```python
from build123d import *

# Parameters (mm, degrees)
SKETCH1_R           = 3.175
BOSS_EXTRUDE1_DEPTH = 2.54


with BuildPart() as part:
    # Sketch1 → Boss-Extrude1 (new body)
    with BuildSketch(Plane.XY):
        with BuildLine():
            Line((-0.792713517, -6.209589215), (80.497230298, -16.587028851))
            Line((80.497230298, -16.587028851), (106.74595178, -3.93139528))
            Line((106.74595178, -3.93139528), (106.274352446, 204.184578368))
            ThreePointArc((106.274352446, 204.184578368), (100.014368984, 210.444561829), (93.754385523, 204.184578368))
            Line((93.754385523, 204.184578368), (94.208186896, 3.92281412))
            Line((94.208186896, 3.92281412), (78.402076612, -3.697989053))
            Line((78.402076612, -3.697989053), (0.792713517, 6.209589215))
            ThreePointArc((0.792713517, 6.209589215), (-6.209589215, 0.792713517), (-0.792713517, -6.209589215))
        make_face()
        Circle(SKETCH1_R, mode=Mode.SUBTRACT)
        with Locations((100.014368984, 204.184578368)):
            Circle(SKETCH1_R, mode=Mode.SUBTRACT)
    extrude(amount=BOSS_EXTRUDE1_DEPTH)


solid = part.part
```
Source: CAD feature listing. Evaluate the final solid. Frame: model axes, mm. Coordinates: 2 decimals unless noted, no trailing zeros. Order: outer loops, then holes, each group sorted by start corner. A loop starts at its lowest first (then second) coordinate and runs counter-clockwise, first axis right, second up. Notation, with made-up numbers: M 88,-23.75 L 137,-23.75 A11 ccw 137,-13.75 Z; hole C -17.75,51.5 d5. An arc over 180 degrees is marked long. Write each question's results on one line, items separated by ' | '. Start each with the question number.
1) Section query B-B (y = 0). Return the cut outline in (x, z) (1 decimal), plus the area to 3 significant figures.
2) Section query C-C (x = 85.5). Return the cut outline in (y, z), plus the area to 3 significant figures.
3) Contact query for a flat-ended pin moving along its axis: pin 1 Ø1.5 at (x, z) = (17.5, 1) entering from +Y. Output: stop coordinate, or through.
4) Line query: line 1 (Y direction, x = 0, z = 1.45) (3 decimals); line 2 (X direction, y = 199, z = 0.7); line 3 (X direction, y = 13.5, z = 0.7). Output: solid intervals per line, ascending. Write a range as from..to.
5) Section query A-A (z = 1.15). Return the cut outline in (x, y) (3 decimals).
6) Draft query along Y for faces 1 (the face through (39.283, -11.326, 1.252)), 2 (the face through (-0.69, -3.1, 1.25)), 3 (the face through (40.141, 1.186, 1.252)). Return one class per face: released by +Y, released by -Y, zero draft, split by the parting line, or undercut.
7) Section query D-D (y = 172). Return the cut outline in (x, z).
Answers:
1) outline: M -6.3,0 L -3.2,0 L -3.2,2.5 L -6.3,2.5 Z; M 3.2,0 L 49.4,0 L 49.4,2.5 L 3.2,2.5 Z; M 86.1,0 L 106.7,0 L 106.7,2.5 L 86.1,2.5 Z | area: 178 mm^2
2) outline: M -14.17,0 L -0.28,0 L -0.28,2.54 L -14.17,2.54 Z | area: 35.3 mm^2
3) pin 1: stops at y = 4.17
4) line 1: y = -6.311..-3.175, 3.175..6.26 | line 2: x = 93.77..106.29 | line 3: x = 94.19..106.71
5) outline: M -0.793,-6.21 L 80.497,-16.587 L 106.746,-3.931 L 106.274,204.185 A6.26 ccw 93.754,204.185 L 94.208,3.923 L 78.402,-3.698 L 0.793,6.21 A6.26 ccw Z; hole C 0,0 d6.35; hole C 100.014,204.185 d6.35
6) face 1: released by -Y | face 2: undercut | face 3: released by +Y
7) outline: M 93.83,0 L 106.35,0 L 106.35,2.54 L 93.83,2.54 Z
